```python
from build123d import *

# Parameters (mm, degrees)
F0_R     = 19
F1_DEPTH = 57
F2_DEPTH = 10
F0_R_2   = 9.5
F3_DEPTH = 38
F5_DEPTH = 57
F7_DEPTH = 36.501


with BuildPart() as f1:
    # F0 (on Top) → F1 (new body)
    with BuildSketch(Plane.XY):
        with BuildLine():
            ThreePointArc((-95.8993569198, 5), (-105.4051754039, 22.9328051198), (-123.8763790613, 31.3447442521))
            ThreePointArc((-123.8763790613, 31.3447442521), (-158.499997838, 0.011670713), (-123.8996062992, -31.3470502424))
            ThreePointArc((-123.8996062992, -31.3470502424), (-105.4136734635, -22.940804403), (-95.8993569198, -5))
            ThreePointArc((-95.8993569198, -5), (-95.5999979536, -2.50796162), (-95.5, 0))
            ThreePointArc((-95.5, 0), (-95.5999979536, 2.50796162), (-95.8993569198, 5))
        make_face()
        with Locations((-127, 0)):
            Circle(F0_R, mode=Mode.SUBTRACT)
    extrude(amount=F1_DEPTH)

    # F0 (on Top) → F2 (join)
    with BuildSketch(Plane.XY):
        with BuildLine():
            Line((-123.8996062992, -31.3470502424), (1.8700787402, -18.9077445907))
            ThreePointArc((1.8700787402, -18.9077445907), (-10.7745572419, -15.6495660081), (-18.3303027798, -5))
            Line((-18.3303027798, -5), (-95.8993569198, -5))
            ThreePointArc((-95.8993569198, -5), (-105.4136734635, -22.940804403), (-123.8996062992, -31.3470502424))
        make_face()
        with BuildLine():
            ThreePointArc((-18.3303027798, 5), (-11.5325625947, 15.0996688705), (0, 19))
            Line((0, 19), (-123.8763790613, 31.3447442521))
            ThreePointArc((-123.8763790613, 31.3447442521), (-105.4051754039, 22.9328051198), (-95.8993569198, 5))
            Line((-95.8993569198, 5), (-18.3303027798, 5))
        make_face()
    extrude(amount=F2_DEPTH)

    # F0 (on Top) → F3 (join)
    with BuildSketch(Plane.XY):
        with BuildLine():
            ThreePointArc((1.8700787402, -18.9077445907), (14.0806870582, -12.7567335932), (19, 0))
            ThreePointArc((19, 0), (13.4350288425, 13.4350288425), (0, 19))
            ThreePointArc((0, 19), (-11.5325625947, 15.0996688705), (-18.3303027798, 5))
            ThreePointArc((-18.3303027798, 5), (-19, 0), (-18.3303027798, -5))
            ThreePointArc((-18.3303027798, -5), (-10.7745572419, -15.6495660081), (1.8700787402, -18.9077445907))
        make_face()
        Circle(F0_R_2, mode=Mode.SUBTRACT)
    extrude(amount=F3_DEPTH)

    # F0 (on Top) → F5 (join)
    with BuildSketch(Plane.XY):
        with BuildLine():
            ThreePointArc((-18.3303027798, -5), (-19, 0), (-18.3303027798, 5))
            Line((-18.3303027798, 5), (-95.8993569198, 5))
            ThreePointArc((-95.8993569198, 5), (-95.5999979536, 2.50796162), (-95.5, 0))
            ThreePointArc((-95.5, 0), (-95.5999979536, -2.50796162), (-95.8993569198, -5))
            Line((-95.8993569198, -5), (-18.3303027798, -5))
        make_face()
    extrude(amount=F5_DEPTH)

    # F6 (on face) → F7 (cut, through all)
    with BuildSketch(Plane.XZ.offset(5)):
        Polygon((-18.3303027798, 57), (-95.8993569198, 57), (-18.3303027798, 38), align=None)
    extrude(amount=-F7_DEPTH, mode=Mode.SUBTRACT)


solid = f1.part
```
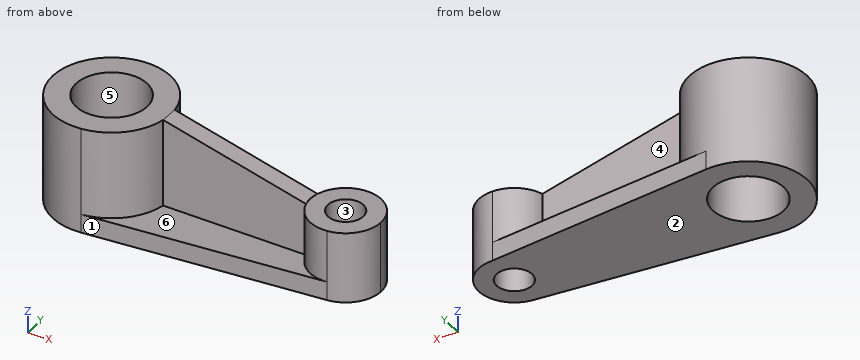
Source: CAD feature listing. Evaluate the final solid. Frame: model axes, mm. Face numbers are marked on the shaded views. A direction names the side the tool comes from. Give positions to 0.01 mm unless a question says otherwise; leave off trailing zeros. Write each loop counter-clockwise with the first axis right and the second up, starting at its lowest first coordinate (ties: lowest second). Pieces come first, ordered by that corner, then holes. Notation, with made-up numbers: (17, 60.25) - (54, 60.25) arc R19 cw to (54, 85.25) - close; hole circle Ø4 at (41.5, 6). An arc over 180 degrees is marked (long way). One line per item, written item: value. Start each with the question number.
Q1. Section query C-C, the plane y = 14. Return the cut outline in (x, z).
Q2. Set-up query: the marked faces 5 and 6. Return all of +Z, -Z, +X, -X, +Y, -Y with unobstructed straight access to the full face (end or side cutting, diameter ignored); none if empty.
Q3. Material intervals for probe 1 along Y at (x, z) = (0, 10.5); probe 2 along Y at (x, z) = (-127, 29); probe 3 along Z at (x, y) = (-88.5, -10.5), sorted ascending. Write a range as from..to.
Q4. Draft query along Y for the marked faces 1, 2, 3 and 4. Return one class per face: +Y half, -Y half, draft (parallel to the pull), parting line (faces both ways), or undercut.
Q5. Section query B-B, the plane z = 26.5. Return the cut outline in (x, y).
Q6. First-contact query: pin 1 Ø5 at (x, z) = (-73.5, 47.5) entering from -Y; pin 2 Ø4 at (x, z) = (-36.5, 14) entering from +Y; pin 3 Ø8 at (x, z) = (-6, 15) entering from +Y. Flat tips, straight axial feed; report the tip coordinate or a pass-through.
Q7. Section query A-A, the plane x = -127. Return the cut outline in (y, z).
Q8. Section query D-D, the plane z = 44. Return the cut outline in (x, y).
Answer:
1. outline: (-155.22, 0) - (-139.85, 0) - (-139.85, 57) - (-155.22, 57) - close; (-114.15, 0) - (12.85, 0) - (12.85, 38) - (-12.85, 38) - (-12.85, 10) - (-98.78, 10) - (-98.78, 57) - (-114.15, 57) - close
2. face 5: +Z, -Z
2. face 6: +Z, -Y
3. probe 1: y = -19..-9.5, 9.5..19
3. probe 2: y = -31.5..-19, 19..31.5
3. probe 3: z = 0..10
4. face 1: -Y half
4. face 2: draft
4. face 3: undercut
4. face 4: +Y half
5. outline: (-95.9, -5) - (-18.33, -5) arc R19 ccw (long way) to (-18.33, 5) - (-95.9, 5) arc R31.5 ccw (long way) to start; hole circle Ø38 at (-127, 0); hole circle Ø19 at (0, 0)
6. pin 1: stops at y = -5
6. pin 2: stops at y = 5
6. pin 3: stops at y = 18.89
7. outline: (-31.5, 0) - (-19, 0) - (-19, 57) - (-31.5, 57) - close; (19, 0) - (31.5, 0) - (31.5, 57) - (19, 57) - close
8. outline: (-95.9, -5) - (-42.83, -5) - (-42.83, 5) - (-95.9, 5) arc R31.5 ccw (long way) to start; hole circle Ø38 at (-127, 0)
